For this review, take the finished solid that the model builds, in its own axes (mm). Face numbers are marked on the shaded views. A direction names the side the tool comes from. Coordinates: 2 decimals unless noted, no trailing zeros. Order: outer loops, then holes, each group sorted by start corner. A loop starts at its lowest first (then second) coordinate and runs counter-clockwise, first axis right, second up. Notation, with made-up numbers: (59, 39.5) - (91, 39.5) arc R4 cw to (91, 44.5) - close; hole circle Ø10 at (81.25, 7). An arc over 180 degrees is marked (long way). One line per item, written item: value. Start each with the question number.
(1) Consider section A-A on z = 24.5. Write out the cut boundary in (x, y).
(2) To check wall thickness, follow line 1 along X through (y, z) = (11, 62); line 2 along Y through (x, z) = (-19, 71.5); line 3 along Z through (x, y) = (-19, -12). State the ranges of each line that lie inside material, in increasing order.
(3) Mouldability with a two-part tool opening along X and no side actions: class the marked faces 3, 4 and 5 as released by +X, released by -X, zero draft, split by the parting line, or undercut.
(4) Clearance check with flat-ended pins moving along their axes: pin 1 (4 mm diameter, centred on x = 13.33, y = 11.89, fed in from +Z); pin 2 (5 mm diameter, centred on x = 22, z = 17.5, fed in from +Y). State where each tip first meets the part, or that it passes through.
(5) For the marked faces 1 and 2, list the 3-axis set-ups (+Z, -Z, +X, -X, +Y, -Y) from which the entire face can be reached by the end or side of a thin tool; tool diameter is ignored.
```python
from build123d import *

# Parameters (mm, degrees)
F0_W         = 50.8
F0_H         = 50.8
F0_R         = 1.5875
F1_DEPTH     = 5.08
F0_W_2       = 55.88
F0_H_2       = 55.88
F2_DEPTH     = 76.2
F3_T1_DEPTH  = 50.8
F4_T4_DEPTH  = 64.3399164321
F4_S5_R      = 5.0800000001
F4_T6_DEPTH  = 34
F5_T4_DEPTH  = 64.3391166785
F5_S5_R      = 5.0813656856
F5_T6_DEPTH  = 34
F6_T4_DEPTH  = 77.8762455026
F6_S6_R      = 5.0800000001
F6_T7_DEPTH  = 41
F6_T11_DEPTH = 77.8762455026
F6_S13_R     = 5.081365685
F6_T14_DEPTH = 41
F7_R         = 5.7567075364
F8_DEPTH     = 8.128
F9_R         = 5.08


# Not quite as in the source:
# - a fillet or chamfer that OpenCascade refuses, or shapes differently, is made with other operations: its cross-section is extruded or revolved along the edge and cut away or added


with BuildPart() as f1:
    # F0 (on Top) → F1 (new body)
    with BuildSketch(Plane.XY):
        with Locations((0.627800245, -0.8074334759)):
            Rectangle(F0_W, F0_H)
        with Locations((-12.072199755, -13.5074334759)):
            Circle(F0_R, mode=Mode.SUBTRACT)
        with Locations((13.327800245, -13.5074334759)):
            Circle(F0_R, mode=Mode.SUBTRACT)
        with Locations((-12.072199755, 11.8925665241)):
            Circle(F0_R, mode=Mode.SUBTRACT)
        with Locations((13.327800245, 11.8925665241)):
            Circle(F0_R, mode=Mode.SUBTRACT)
    extrude(amount=F1_DEPTH)

    # F0 (on Top) → F2 (join)
    with BuildSketch(Plane.XY):
        with Locations((0.627800245, -0.8074334759)):
            Rectangle(F0_W_2, F0_H_2)
        with Locations((0.627800245, -0.8074334759)):
            Rectangle(F0_W, F0_H, mode=Mode.SUBTRACT)
    extrude(amount=F2_DEPTH)

    # F3: fillet of radius 5.08 on 1 edges, made by hand

    # F3_s2 → F3_t1 (cut)
    with BuildSketch(Plane.YZ.offset(-24.772199755)):
        with BuildLine():
            ThreePointArc((-26.2074334759, 71.12), (-27.6953310275, 74.7121024484), (-31.2874334759, 76.2))
            Line((-31.2874334759, 76.2), (-26.2074334759, 76.2))
            Line((-26.2074334759, 76.2), (-26.2074334759, 71.12))
        make_face()
    extrude(amount=F3_T1_DEPTH, mode=Mode.SUBTRACT)

    # F4: fillet of radius 5.08 on 1 edges, made by hand


with BuildPart() as f4_tool2:
    # F4_s3 → F4_t4 (new body)
    with BuildSketch(Plane.XZ.offset(-24.5925665241)):
        with BuildLine():
            ThreePointArc((-27.311999717, 76.2003463882), (-25.4524342775, 74.3404748362), (-24.771799755, 71.8000334454))
            Line((-24.771799755, 71.8000334454), (-24.2636631865, 71.8000334454))
            ThreePointArc((-24.2636631865, 71.8000334454), (-24.2640631865, 74.0000167227), (-24.2640631865, 76.2))
            Line((-24.2640631865, 76.2), (-24.772199755, 76.7081365685))
            ThreePointArc((-24.772199755, 76.7081365685), (-26.042099736, 76.7081365685), (-27.0578831447, 76.6403776825))
            Line((-27.0578831447, 76.6403776825), (-27.311999717, 76.2003463882))
        make_face()
    extrude(amount=F4_T4_DEPTH)

    # F4_s5 → F4_t6 (cut, symmetric)
    with BuildSketch(Plane.YZ.offset(-25.8)):
        with Locations((-31.287433476, 71.1199999999)):
            Circle(F4_S5_R)
    extrude(amount=F4_T6_DEPTH, both=True, mode=Mode.SUBTRACT)


with BuildPart() as f1_1:
    add(f1.part)

    # F4_t1: cut F4_tool2
    add(f4_tool2.part, mode=Mode.SUBTRACT)

    # F5: fillet of radius 5.08 on 1 edges, made by hand


with BuildPart() as f5_tool2:
    # F5_s3 → F5_t4 (new body)
    with BuildSketch(Plane.YZ.offset(26.027800245)):
        with BuildLine():
            ThreePointArc((24.5921665241, 71.8000334454), (25.2728010465, 74.3404748362), (27.1323664861, 76.2003463882))
            Line((27.1323664861, 76.2003463882), (26.8782499137, 76.6403776825))
            ThreePointArc((26.8782499137, 76.6403776825), (25.8624665051, 76.7081365685), (24.5925665241, 76.7081365685))
            Line((24.5925665241, 76.7081365685), (24.0844299555, 76.2))
            ThreePointArc((24.0844299555, 76.2), (24.0844299555, 74.0000167227), (24.0840299555, 71.8000334454))
            Line((24.0840299555, 71.8000334454), (24.5921665241, 71.8000334454))
        make_face()
    extrude(amount=-F5_T4_DEPTH)

    # F5_s5 → F5_t6 (cut, symmetric)
    with BuildSketch(Plane.XZ.offset(-25.6)):
        with Locations((-29.8531654406, 71.8000334452)):
            Circle(F5_S5_R)
    extrude(amount=F5_T6_DEPTH, both=True, mode=Mode.SUBTRACT)


with BuildPart() as f1_2:
    add(f1_1.part)

    # F5_t1: cut F5_tool2
    add(f5_tool2.part, mode=Mode.SUBTRACT)

    # F6: fillet of radius 5.08 on 1 edges, made by hand


with BuildPart() as f6_tool2:
    # F6_s3 → F6_t4 (new body)
    with BuildSketch(Plane.XZ.offset(39.745956104)):
        with BuildLine():
            ThreePointArc((28.567800245, 76.2), (26.7083911938, 74.3405909488), (26.027800245, 71.8005909488))
            Line((26.027800245, 71.8005909488), (26.027800245, 76.2))
            Line((26.027800245, 76.2), (28.567800245, 76.2))
        make_face()
    extrude(amount=-F6_T4_DEPTH)

    split(bisect_by=Plane.XZ.offset(-24.5925665241), keep=Keep.TOP)

    # F6_s6 → F6_t7 (cut, symmetric)
    with BuildSketch(Plane.YZ.offset(27.3)):
        with Locations((-31.287433476, 71.1199999999)):
            Circle(F6_S6_R)
    extrude(amount=F6_T7_DEPTH, both=True, mode=Mode.SUBTRACT)


with BuildPart() as f1_3:
    add(f1_2.part)

    # F6_t1: cut F6_tool2
    add(f6_tool2.part, mode=Mode.SUBTRACT)


with BuildPart() as f6_tool9:
    # F6_s10 → F6_t11 (new body)
    with BuildSketch(Plane.XZ.offset(39.745956104)):
        with BuildLine():
            ThreePointArc((28.567800245, 76.2), (26.7083911938, 74.3405909488), (26.027800245, 71.8005909488))
            Line((26.027800245, 71.8005909488), (26.027800245, 76.2))
            Line((26.027800245, 76.2), (28.567800245, 76.2))
        make_face()
    extrude(amount=-F6_T11_DEPTH)

    split(bisect_by=Plane.XZ.offset(-24.5925665241), keep=Keep.BOTTOM)

    # F6_s13 → F6_t14 (cut, symmetric)
    with BuildSketch(Plane.YZ.offset(27.3)):
        with Locations((29.6735322091, 71.8000334456)):
            Circle(F6_S13_R)
    extrude(amount=F6_T14_DEPTH, both=True, mode=Mode.SUBTRACT)


with BuildPart() as f1_4:
    add(f1_3.part)

    # F6_t8: cut F6_tool9
    add(f6_tool9.part, mode=Mode.SUBTRACT)

    # F7 (on face) → F8 (join)
    with BuildSketch(Plane(origin=(0, 27.1325665241, 0), x_dir=(-1, 0, 0), z_dir=(0, 1, 0))):
        with Locations((0, 38.1)):
            Circle(F7_R)
    extrude(amount=F8_DEPTH)

    # F9
    f9_edges = [f1_4.edges().sort_by_distance(p)[0] for p in [
        (5.756708, 35.260567, 38.1),
    ]]
    fillet(f9_edges, radius=F9_R)


solid = f1_4.part
```
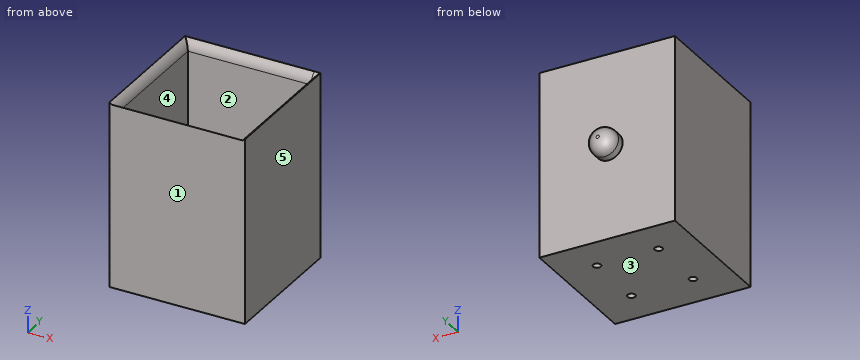
Geometry check:
1. outline: (-27.31, -28.75) - (28.57, -28.75) - (28.57, 27.13) - (-27.31, 27.13) - close; hole (-24.77, -26.21) - (26.03, -26.21) - (26.03, 24.59) - (-24.77, 24.59) - close
2. line 1: x = -27.31 to -24.77, 26.03 to 28.57
2. line 2: y = -28.75 to -26.22, 24.59 to 27.13
2. line 3: z = 0 to 5.08
3. face 3: zero draft
3. face 4: undercut
3. face 5: released by +X
4. pin 1: stops at z = 5.08
4. pin 2: stops at y = 27.13
5. face 1: +Z, -Z, +X, -X, -Y
5. face 2: +Z
